```python
from build123d import *

# Parameters (mm, degrees)
SKETCH1_W             = 23
SKETCH1_H             = 23
BOSS_EXTRUDE1_DEPTH   = 2
FILLET1_R             = 2
SKETCH2_R             = 1.6
CUT_EXTRUDE1_DEPTH    = 2
SKETCH3_W             = 10.8
SKETCH3_H             = 2.3
CUT_EXTRUDE2_DEPTH    = 2
SKETCH5_R             = 1.6
BOSS_EXTRUDE2_DEPTH   = 2
BOSS_EXTRUDE2_2_DEPTH = 2
BOSS_EXTRUDE2_3_DEPTH = 2
BOSS_EXTRUDE2_4_DEPTH = 2
BOSS_EXTRUDE3_START   = 2
SKETCH6_R             = 3.1
SKETCH6_R_2           = 1.6
BOSS_EXTRUDE3_DEPTH   = 1.1


with BuildPart() as part:
    # Sketch1 → Boss-Extrude1 (new body)
    with BuildSketch(Plane.XY):
        with Locations((11.5, 11.5)):
            Rectangle(SKETCH1_W, SKETCH1_H)
    extrude(amount=BOSS_EXTRUDE1_DEPTH)

    # Fillet1
    fillet1_edges = [part.edges().sort_by_distance(p)[0] for p in [
        (0, 23, 1),
        (23, 23, 1),
        (23, 0, 1),
        (0, 0, 1),
    ]]
    fillet(fillet1_edges, radius=FILLET1_R)

    # Sketch2 → Cut-Extrude1 (cut)
    with BuildSketch(Plane.XY):
        with Locations((3.5, 19.7)):
            Circle(SKETCH2_R)
        with Locations((19.5, 19.7)):
            Circle(SKETCH2_R)
        with Locations((19.5, 3.5)):
            Circle(SKETCH2_R)
        with Locations((3.5, 3.5)):
            Circle(SKETCH2_R)
        with BuildLine():
            Line((3.5, 17.1), (3.5, 6.1))
            ThreePointArc((3.5, 6.1), (5.338477631, 5.338477631), (6.1, 3.5))
            Line((6.1, 3.5), (16.9, 3.5))
            ThreePointArc((16.9, 3.5), (17.661522369, 5.338477631), (19.5, 6.1))
            Line((19.5, 6.1), (19.5, 17.1))
            ThreePointArc((19.5, 17.1), (17.661522369, 17.861522369), (16.9, 19.7))
            Line((16.9, 19.7), (6.1, 19.7))
            ThreePointArc((6.1, 19.7), (5.338477631, 17.861522369), (3.5, 17.1))
        make_face()
    extrude(amount=CUT_EXTRUDE1_DEPTH, mode=Mode.SUBTRACT)

    # Sketch3 → Cut-Extrude2 (cut)
    with BuildSketch(Plane.XY):
        with Locations((11.5, 20.85)):
            Rectangle(SKETCH3_W, SKETCH3_H)
    extrude(amount=CUT_EXTRUDE2_DEPTH, mode=Mode.SUBTRACT)


with BuildPart() as body_2:
    # Sketch5 → Boss-Extrude2 (new body)
    with BuildSketch(Plane.XY):
        with BuildLine():
            Line((16.9, 23), (21.776453683, 21.561960094))
            Line((21.776453683, 21.561960094), (23, 12.648059803))
            ThreePointArc((23, 12.648059803), (23.313519219, 13.886650017), (24.17856315, 14.826915413))
            Line((24.17856315, 14.826915413), (29.65108056, 18.405475842))
            ThreePointArc((29.65108056, 18.405475842), (30.877170115, 22.033391556), (27.643175365, 24.084329386))
            Line((27.643175365, 24.084329386), (16.9, 23))
        make_face()
        with Locations((27.954482672, 21)):
            Circle(SKETCH5_R, mode=Mode.SUBTRACT)
    extrude(amount=BOSS_EXTRUDE2_DEPTH)


with BuildPart() as body_3:
    # Sketch5 → Boss-Extrude2 2 (new body)
    with BuildSketch(Plane.XY):
        with BuildLine():
            Line((-4.643175365, 24.084329386), (6.1, 23))
            Line((6.1, 23), (1.223546317, 21.561960094))
            Line((1.223546317, 21.561960094), (0, 12.648059803))
            ThreePointArc((0, 12.648059803), (-0.313519219, 13.886650017), (-1.17856315, 14.826915413))
            Line((-1.17856315, 14.826915413), (-6.65108056, 18.405475842))
            ThreePointArc((-6.65108056, 18.405475842), (-7.877170115, 22.033391556), (-4.643175365, 24.084329386))
        make_face()
        with Locations((-4.954482672, 21)):
            Circle(SKETCH5_R, mode=Mode.SUBTRACT)
    extrude(amount=BOSS_EXTRUDE2_2_DEPTH)


with BuildPart() as body_4:
    # Sketch5 → Boss-Extrude2 3 (new body)
    with BuildSketch(Plane.XY):
        with BuildLine():
            Line((16.9, 0), (21.776453683, 1.438039906))
            Line((21.776453683, 1.438039906), (23, 10.351940197))
            ThreePointArc((23, 10.351940197), (23.313519219, 9.113349983), (24.17856315, 8.173084587))
            Line((24.17856315, 8.173084587), (29.65108056, 4.594524158))
            ThreePointArc((29.65108056, 4.594524158), (30.877170115, 0.966608444), (27.643175365, -1.084329386))
            Line((27.643175365, -1.084329386), (16.9, 0))
        make_face()
        with Locations((27.954482672, 2)):
            Circle(SKETCH5_R, mode=Mode.SUBTRACT)
    extrude(amount=BOSS_EXTRUDE2_3_DEPTH)


with BuildPart() as body_5:
    # Sketch5 → Boss-Extrude2 4 (new body)
    with BuildSketch(Plane.XY):
        with BuildLine():
            Line((6.1, 0), (1.223546317, 1.438039906))
            Line((1.223546317, 1.438039906), (0, 10.351940197))
            ThreePointArc((0, 10.351940197), (-0.313519219, 9.113349983), (-1.17856315, 8.173084587))
            Line((-1.17856315, 8.173084587), (-6.65108056, 4.594524158))
            ThreePointArc((-6.65108056, 4.594524158), (-7.877170115, 0.966608444), (-4.643175365, -1.084329386))
            Line((-4.643175365, -1.084329386), (6.1, 0))
        make_face()
        with Locations((-4.954482672, 2)):
            Circle(SKETCH5_R, mode=Mode.SUBTRACT)
    extrude(amount=BOSS_EXTRUDE2_4_DEPTH)

    # Combine1: union part, body 3, body 2, body 4
    add(part.part)
    add(body_3.part)
    add(body_2.part)
    add(body_4.part)

    # Sketch6 → Boss-Extrude3 (add)
    with BuildSketch(Plane.XY.offset(BOSS_EXTRUDE3_START)):
        with Locations((-4.954482672, 21)):
            Circle(SKETCH6_R)
        with Locations((-4.954482672, 21)):
            Circle(SKETCH6_R_2, mode=Mode.SUBTRACT)
        with Locations((-4.954482672, 2)):
            Circle(SKETCH6_R)
        with Locations((-4.954482672, 2)):
            Circle(SKETCH6_R_2, mode=Mode.SUBTRACT)
        with Locations((27.954482672, 2)):
            Circle(SKETCH6_R)
        with Locations((27.954482672, 2)):
            Circle(SKETCH6_R_2, mode=Mode.SUBTRACT)
        with Locations((27.954482672, 21)):
            Circle(SKETCH6_R)
        with Locations((27.954482672, 21)):
            Circle(SKETCH6_R_2, mode=Mode.SUBTRACT)
    extrude(amount=BOSS_EXTRUDE3_DEPTH)


solid = body_5.part
```
Verification items for the finished model (mm, model axes). A direction names the side the tool comes from. Give positions to 0.01 mm unless a question says otherwise; leave off trailing zeros. Loops run counter-clockwise (first coordinate to the right, second up) from the corner with the lowest first, then second, coordinate; pieces in that order, holes last.
1. Thickness scan on line 1 (Y direction, x = 10, z = 1.9); line 2 (Y direction, x = -5.5, z = 0.4); line 3 (X direction, y = 4.5, z = 2.75). Record the ranges inside material, lowest first.
2. Set-up check for faces 1 (the flat face through (26.877, 6.409, 0.986)), 2 (the flat face through (0, 11, 1)), 3 (the flat face through (22.35, -0.55, 0.99)), 4 (the flat face through (22.35, 23.55, 0.99)): record each of +Z, -Z, +X, -X, +Y, -Y from which the full face is reachable in a straight line by a thin tool's end or side.
3. Go/stop test with flat-tipped pins: pin 1 Ø3.5 at (x, y) = (3.5, 19.7) entering from +Z; pin 2 Ø3 at (x, y) = (19.5, 19.7) entering from -Z; pin 3 Ø1.6 at (x, z) = (12.5, 0.5) entering from +Y; pin 4 Ø1 at (x, z) = (-1.5, 2) entering from -Y. Record where each tip stops, or that it passes through.
4. Mould release check, pull along Y, two halves, no side actions. Record for faces 5 (the flat face through (-3.877, 16.591, 0.986)), 6 (the flat face through (-3.6, 0.7, 3.1)), 7 (the flat face through (0.65, 23.55, 0.99)): released by +Y, released by -Y, zero draft, split by the parting line, or undercut.
5. Section check A-A, the plane x = 7. Enter the section's corners in (y, z), then the cut area to 3 significant figures.
6. Section check B-B, the plane z = 2.5. Enter the section's corners in (x, y), then the cut area to 3 significant figures.
7. Section check C-C, the plane y = 10.75. Enter the section's corners in (x, z).
8. Section check D-D, the plane x = 3. Enter the section's corners in (y, z), then the cut area to 3 significant figures.
Geometry says:
1. line 1: y = 0 to 3.5, 22 to 23
1. line 2: y = -1.05 to 0.5, 3.5 to 5.35, 17.65 to 19.5, 22.5 to 24.05
1. line 3: x = -6.79 to -3.12, 26.12 to 29.79
2. face 1: +Z, -Z, +X
2. face 2: +Z, -Z, -X
2. face 3: +Z, -Z, -Y
2. face 4: +Z, -Z, +Y
3. pin 1: stops at z = 2
3. pin 2: passes through
3. pin 3: stops at y = 23
3. pin 4: stops at y = -0.82
4. face 5: undercut
4. face 6: zero draft
4. face 7: released by +Y
5. outline: (0, 0) - (3.5, 0) - (3.5, 2) - (0, 2) - close; (22, 0) - (23, 0) - (23, 2) - (22, 2) - close
5. area: 9.00 mm2
6. outline: circle Ø6.2 at (-4.95, 2); circle Ø6.2 at (-4.95, 21); circle Ø6.2 at (27.95, 2); circle Ø6.2 at (27.95, 21); hole circle Ø3.2 at (-4.95, 2); hole circle Ø3.2 at (-4.95, 21); hole circle Ø3.2 at (27.95, 2); hole circle Ø3.2 at (27.95, 21)
6. area: 88.6 mm2
7. outline: (0, 0) - (3.5, 0) - (3.5, 2) - (0, 2) - close; (19.5, 0) - (23, 0) - (23, 2) - (19.5, 2) - close
8. outline: (-0.31, 0) - (1.98, 0) - (1.98, 2) - (-0.31, 2) - close; (5.02, 0) - (18.18, 0) - (18.18, 2) - (5.02, 2) - close; (21.22, 0) - (23.31, 0) - (23.31, 2) - (21.22, 2) - close
8. area: 35.1 mm2
